Could you check a few things on this model? Use its own coordinates, in mm. A direction names the side the tool comes from. Give positions to 0.01 mm unless a question says otherwise; leave off trailing zeros. Order: outer loops, then holes, each group sorted by start corner. A loop starts at its lowest first (then second) coordinate and runs counter-clockwise, first axis right, second up. Notation, with made-up numbers: M 16.5,61 L 70.5,61 A24 ccw 70.5,74 Z; hole C -6,-33.5 d10. An arc over 180 degrees is marked long. Answer in a Markdown table with one row per item. Add a question column.
```python
from build123d import *

# Parameters (mm, degrees)
SKETCH1_R           = 1.5
BOSS_EXTRUDE1_DEPTH = 6
BOSS_EXTRUDE2_DEPTH = 1


with BuildPart() as part:
    # Sketch1 → Boss-Extrude1 (new body)
    with BuildSketch(Plane(origin=(0, 0, 0), x_dir=(1, 0, 0), z_dir=(0, 1, 0))):
        with BuildLine():
            ThreePointArc((2.346955398, 0.261158526), (0.766582759, -0.648437779), (0.581159215, -2.462428195))
            Line((0.581159215, -2.462428195), (-5.646281291, -5.138082195))
            Line((-5.646281291, -5.138082195), (-6.527676066, -12.586111683))
            Line((-6.527676066, -12.586111683), (-0.518190709, -17.073436693))
            Line((-0.518190709, -17.073436693), (4.364038924, -14.975759929))
            Line((4.364038924, -14.975759929), (2.260805866, -7.930513525))
            Line((2.260805866, -7.930513525), (15.112004176, -2.408925622))
            Line((15.112004176, -2.408925622), (15.993398951, 5.039103866))
            Line((15.993398951, 5.039103866), (9.983913594, 9.526428876))
            Line((9.983913594, 9.526428876), (3.093033462, 6.565724398))
            Line((3.093033462, 6.565724398), (2.346955398, 0.261158526))
        make_face()
        with Locations((2.445675843, -1.738841474)):
            Circle(SKETCH1_R, mode=Mode.SUBTRACT)
    extrude(amount=BOSS_EXTRUDE1_DEPTH)

    # Sketch2 → Boss-Extrude2 (add)
    with BuildSketch(Plane(origin=(0, 6, 0), x_dir=(1, 0, 0), z_dir=(0, 1, 0))):
        with BuildLine():
            Line((0.469627416, -1.421953369), (-6.571502088, -4.447213314))
            Line((-6.571502088, -4.447213314), (-7.588596466, -13.041941957))
            Line((-7.588596466, -13.041941957), (-0.653890312, -18.220135847))
            Line((-0.653890312, -18.220135847), (7.29791022, -14.803601096))
            Line((7.29791022, -14.803601096), (8.288969653, -6.428874937))
            Line((8.288969653, -6.428874937), (16.037224973, -3.099794503))
            Line((16.037224973, -3.099794503), (17.054319351, 5.494934139))
            Line((17.054319351, 5.494934139), (10.119613197, 10.67312803))
            Line((10.119613197, 10.67312803), (2.167812665, 7.256593278))
            Line((2.167812665, 7.256593278), (1.297445688, -0.098248268))
            ThreePointArc((1.297445688, -0.098248268), (1.796782906, 0.15567759), (2.346955398, 0.261158526))
            Line((2.346955398, 0.261158526), (3.093033462, 6.565724398))
            Line((3.093033462, 6.565724398), (9.983913594, 9.526428876))
            Line((9.983913594, 9.526428876), (15.993398951, 5.039103866))
            Line((15.993398951, 5.039103866), (15.112004176, -2.408925622))
            Line((15.112004176, -2.408925622), (2.260805866, -7.930513525))
            Line((2.260805866, -7.930513525), (4.364038924, -14.975759929))
            Line((4.364038924, -14.975759929), (-0.518190709, -17.073436693))
            Line((-0.518190709, -17.073436693), (-6.527676066, -12.586111683))
            Line((-6.527676066, -12.586111683), (-5.646281291, -5.138082195))
            Line((-5.646281291, -5.138082195), (0.581159215, -2.462428195))
            ThreePointArc((0.581159215, -2.462428195), (0.456138011, -1.949614478), (0.469627416, -1.421953369))
        make_face()
    extrude(amount=-BOSS_EXTRUDE2_DEPTH)


solid = part.part
```
1. Suppose I cut it at C-C on x = 10.5. List the corners of the cut face in (y, z) for me.
2. Suppose I cut it at B-B on z = 12. List the corners of the cut face in (x, y) for me, plus the area to 3 significant figures.
3. Thinking about a two-plate mould opening in X: for faces 6 (the flat face through (12.109, 5.507, 4.788)), 7 (the flat face through (6.2, 5.51, -8.99)), 8 (the cylindrical face through (3.14, 2.96, 3.07)), 9 (the flat face through (5, 5, 7)), which applies, pulls with the +X half, pulls with the -X half, needs draft (parallel to the pull), parting line crosses it, or undercut?
4. Will these pins go through, and if not, where does the flat tip stop? P1, Ø4, axis at x = 9, z = 3.5, coming from the -Y side; P2, Ø2, axis at y = 5, z = 8.5, coming from the +X side; P3, Ø2, axis at x = -3.5, y = 1, coming from the +Z side; P4, Ø1.5, axis at y = 1.5, z = -2.5, coming from the -X side.
5. Suppose I cut it at A-A on y = 3.6. List the corners of the cut face in (x, z) for me.
6. Suppose I cut it at D-D on y = 5.5. List the corners of the cut face in (x, z) for me.
7. For faces 1 (the cylindrical face through (0.8, 3, 0.6)), 2 (the flat face through (15.547, 2.465, -1.263)), 3 (the flat face through (6.59, 2.46, -8.07)), 4 (the flat face through (1.74, 5.51, -3.63)), 5 (the flat face through (8.596, 2.465, 5.208)), which set-ups out of +Z, -Z, +X, -X, +Y, -Y let a thin tool reach every point of the face, with its end or its side?
8. If I drill on line 1 along X through (y, z) = (3.25, 2.5); line 2 along Z through (x, y) = (1.25, 4.85); line 3 along Z through (x, y) = (8, 4.35), over which ranges is the centre line in solid material (lowest first)? Write a range as [from, to].
Findings below:
| question | item | result |
|---|---|---|
| 1 | outline | M 0,-9.14 L 5,-9.14 L 5,-10.39 L 6,-10.39 L 6,5.48 L 5,5.48 L 5,4.39 L 0,4.39 Z |
| 2 | outline | M -7.47,5 L -6.46,5 L -6.46,0 L 3.48,0 L 3.48,5 L 7.63,5 L 7.63,6 L -7.47,6 Z |
| 2 | area | 64.8 mm2 |
| 3 | face 6 | pulls with the +X half |
| 3 | face 7 | pulls with the -X half |
| 3 | face 8 | undercut |
| 3 | face 9 | needs draft |
| 4 | P1 | y = 0 |
| 4 | P2 | x = 8.16 |
| 4 | P3 | z = 15.59 |
| 4 | P4 | x = 2.52 |
| 5 | outline | M -6.53,12.59 L -5.65,5.14 L 0.58,2.46 A2 ccw 2.35,-0.26 L 3.09,-6.57 L 9.98,-9.53 L 15.99,-5.04 L 15.11,2.41 L 2.26,7.93 L 4.36,14.98 L -0.52,17.07 Z; hole C 2.45,1.74 d3 |
| 6 | outline | M -7.59,13.04 L -6.57,4.45 L 0.47,1.42 A2 ccw 1.3,0.1 L 2.17,-7.26 L 10.12,-10.67 L 17.05,-5.49 L 16.04,3.1 L 8.29,6.43 L 7.3,14.8 L -0.65,18.22 Z; hole C 2.45,1.74 d3 |
| 7 | face 1 | -X, -Y |
| 7 | face 2 | +Z, +X, -Y |
| 7 | face 3 | -Z, -X, -Y |
| 7 | face 4 | -Z, -X, +Y, -Y |
| 7 | face 5 | +X, -Y |
| 8 | line 1 | [0.49, 1.15], [3.74, 14.9] |
| 8 | line 2 | [0.13, 0.83], [2.64, 16.31] |
| 8 | line 3 | [-8.67, 5.46] |
